Check sheet for the drawn part. Datum: minimum x, y, z corner. Units: mm. A direction names the side the tool comes from. Round coordinates to 2 decimals unless told otherwise and drop trailing zeros. Order: outer loops, then holes, each group sorted by start corner. A loop starts at its lowest first (then second) coordinate and runs counter-clockwise, first axis right, second up. Notation, with made-up numbers: (-4.75, -9.5) -> (18.25, -9.5) arc R24 cw to (18.25, 21.5) -> close; hole circle Ø10 at (77, -19.5). An arc over 180 degrees is marked (long way). Answer in a Markdown table with one row per item.
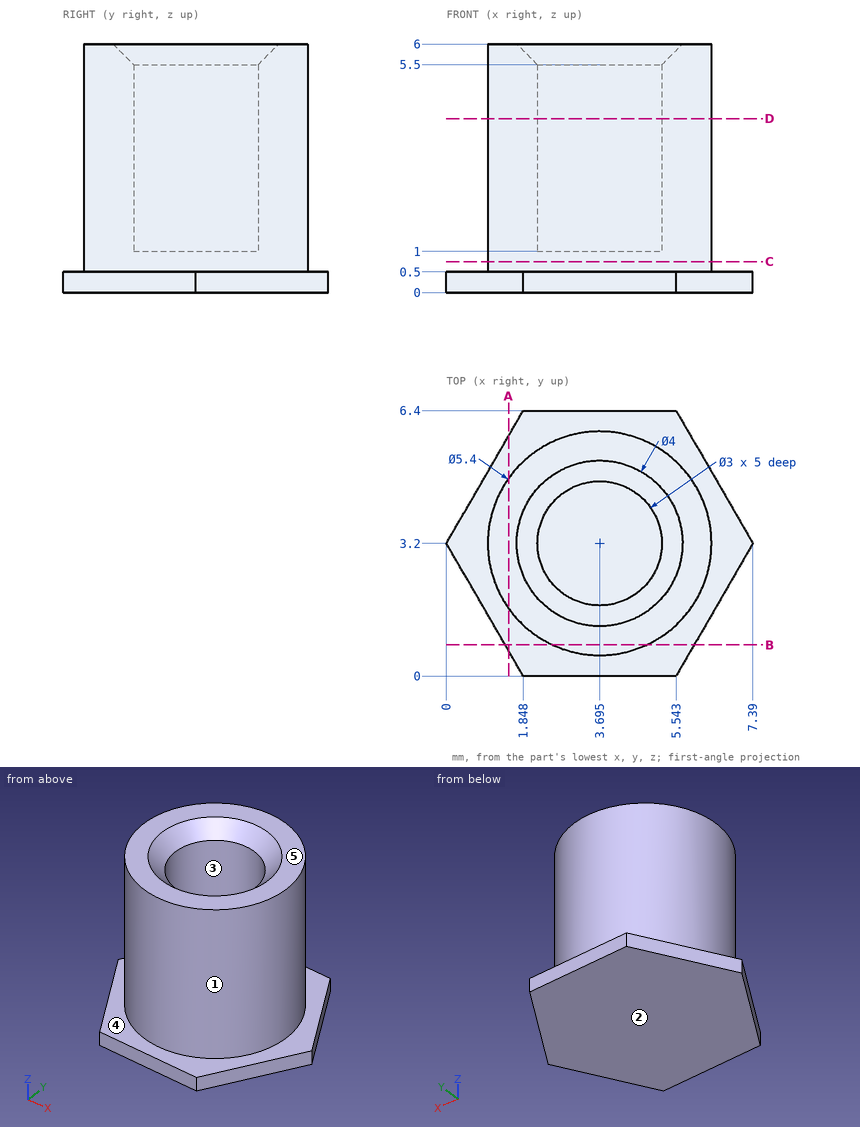
(1) Draft check along X on the marked faces 1, 2 and 3. Enter one of: pulls with the +X half, pulls with the -X half, needs draft (parallel to the pull), parting line crosses it, or undercut.
Solutions:
| item | result |
|---|---|
| face 1 | parting line crosses it |
| face 2 | needs draft |
| face 3 | undercut |
(2) Tool access check on the marked faces 4 and 5. Record the directions out of +Z, -Z, +X, -X, +Y, -Y that give a thin tool (end or side, any length) a straight path to the whole face; none if there is none.
Solutions:
| item | result |
|---|---|
| face 4 | +Z |
| face 5 | +Z, +X, -X, +Y, -Y |
(3) Section check A-A on x = 1.5. Record the boundary of the cut face in (y, z).
Solutions:
| item | result |
|---|---|
| outline | (0.6, 0) -> (5.8, 0) -> (5.8, 0.5) -> (4.77, 0.5) -> (4.77, 6) -> (1.63, 6) -> (1.63, 0.5) -> (0.6, 0.5) -> close |
(4) Section check C-C on z = 0.75. Record the boundary of the cut face in (x, y) (1 decimal), plus the area to 3 significant figures.
Solutions:
| item | result |
|---|---|
| outline | circle Ø5.4 at (3.7, 3.2) |
| area | 22.9 mm^2 |
(5) Section check D-D on z = 4.2. Record the boundary of the cut face in (x, y) (1 decimal).
Solutions:
| item | result |
|---|---|
| outline | circle Ø5.4 at (3.7, 3.2); hole circle Ø3 at (3.7, 3.2) |
(6) Scan lines: probe 1 along Z at (x, y) = (3.5, 3.25); probe 2 along Y at (x, z) = (2.5, 5.4) (1 decimal); probe 3 along Z at (x, y) = (1.75, 5.75). Record each from-to range of solid material in increasing order. Write a range as from..to.
Solutions:
| item | result |
|---|---|
| probe 1 | 0..1 |
| probe 2 | 0.8..2.3, 4.1..5.6 |
| probe 3 | 0..0.5 |
(7) Section check B-B on y = 0.75. Record the boundary of the cut face in (x, z) (1 decimal).
Solutions:
| item | result |
|---|---|
| outline | (1.4, 0) -> (6, 0) -> (6, 0.5) -> (4.8, 0.5) -> (4.8, 6) -> (2.6, 6) -> (2.6, 0.5) -> (1.4, 0.5) -> close |
(8) Depth check by flat-ended pin: pin 1 Ø0.9 at (x, y) = (3.5, 3) entering from +Z; pin 2 Ø3.5 at (x, y) = (3.695, 3.2) entering from +Z; pin 3 Ø1.5 at (x, z) = (6.5, 3.5) entering from -Y. Enter the tip coordinate at first touch or a pass-through.
Solutions:
| item | result |
|---|---|
| pin 1 | z = 1 |
| pin 2 | z = 5.75 |
| pin 3 | y = 1.45 |
